from build123d import *

# Parameters (mm, degrees)
F0_W     = 40
F0_H     = 20
F0_W_2   = 80
F0_H_2   = 100
F0_R     = 5.444049
F0_H_3   = 20.000004
F0_R_2   = 5.262192
F0_R_3   = 5.424143
F1_DEPTH = 25


with BuildPart() as f1:
    # F0 (on Front) → F1 (new body)
    with BuildSketch(Plane.XZ):
        Polygon((-162.994809, -39.040719), (-162.994809, -53.924445), (-42.994809, -53.924445), (-42.994809, -33.45933), (-12.994809, -33.45933), (-12.994809, 66.540668), (-42.994809, 66.540668), (-42.994809, 86.075555), (-162.994809, 86.075555), (-162.994809, 76.773231), (-169.971554, 68.866255), (-212.994809, 68.866255), (-212.994809, -31.133745), (-169.971554, -31.133745), align=None)
        with Locations((-182.994809, -14.622118)):
            Rectangle(F0_W, F0_H, mode=Mode.SUBTRACT)
        with Locations((-104.85527, 13.749972)):
            Rectangle(F0_W_2, F0_H_2, mode=Mode.SUBTRACT)
        with Locations((-28.438857, -9.738397)):
            Circle(F0_R, mode=Mode.SUBTRACT)
        Polygon((-202.994809, 7.936021), (-202.994809, 27.936022), (-175.087825, 27.936022), (-162.994809, 27.936022), (-162.994809, 7.936021), (-175.087825, 7.936021), align=None, mode=Mode.SUBTRACT)
        with Locations((-182.994809, 49.563928)):
            Rectangle(F0_W, F0_H_3, mode=Mode.SUBTRACT)
        with Locations((-28.257, 21.424393)):
            Circle(F0_R_2, mode=Mode.SUBTRACT)
        with Locations((-28.418952, 48.866255)):
            Circle(F0_R_3, mode=Mode.SUBTRACT)
    extrude(amount=F1_DEPTH)


solid = f1.part
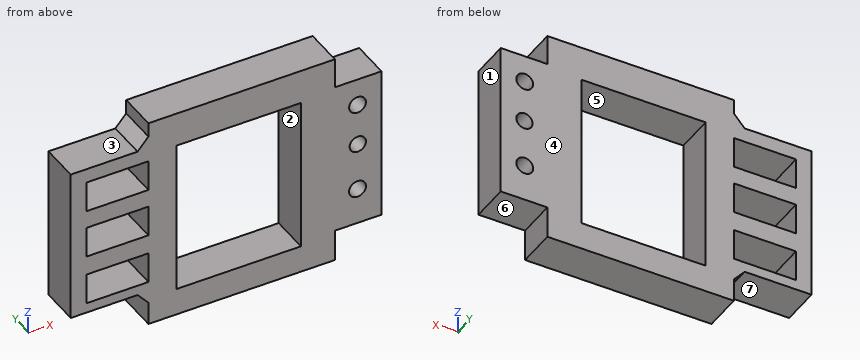
Here's how the part is built. I have some questions about the finished solid (model axes, mm). Face numbers are marked on the shaded views. A direction names the side the tool comes from. Round coordinates to 2 decimals unless told otherwise and drop trailing zeros. Write each loop counter-clockwise with the first axis right and the second up, starting at its lowest first coordinate (ties: lowest second). Pieces come first, ordered by that corner, then holes. Notation, with made-up numbers: (58, -17) -> (69, -17) arc R8 cw to (69, -7) -> close; hole circle Ø6 at (-0.75, 0.25). An arc over 180 degrees is marked (long way). One line per item, written item: value.
1) I'm going to push flat-ended pins straight in: pin 1 Ø7.5 at (x, y) = (-24, -8.5) entering from -Z; pin 2 Ø8 at (x, z) = (-142.5, -21.5) entering from -Y; pin 3 Ø3 at (x, y) = (-166.5, -2.5) entering from +Z; pin 4 Ø12.5 at (x, y) = (-191.5, -17.5) entering from +Z. Where does each tip first touch, or does it pass through?
Filled sheet:
pin 1: stops at z = -33.46
pin 2: stops at y = -25
pin 3: stops at z = 74.5
pin 4: stops at z = 68.87
2) Suppose I cut it at B-B on x = -142. List the corners of the cut face in (y, z) for me.
Filled sheet:
outline: (-25, -53.92) -> (0, -53.92) -> (0, -36.25) -> (-25, -36.25) -> close; (-25, 63.75) -> (0, 63.75) -> (0, 86.08) -> (-25, 86.08) -> close
3) We'd pull the mould along Z, two halves only. Please class the marked faces 1, 2 and 3: released by +Z, released by -Z, zero draft, split by the parting line, or undercut.
Filled sheet:
face 1: zero draft
face 2: undercut
face 3: released by +Z
4) If I drill on line 1 (X direction, y = -3.25, z = 13); line 2 (X direction, y = -8.5, z = 21.5); line 3 (Z direction, x = -199, y = -13), over which ranges is the centre line in solid material (lowest first)? Write a range as [from, to].
Filled sheet:
line 1: x = [-212.99, -202.99], [-162.99, -144.86], [-64.86, -12.99]
line 2: x = [-212.99, -202.99], [-162.99, -144.86], [-64.86, -33.52], [-23, -12.99]
line 3: z = [-31.13, -24.62], [-4.62, 7.94], [27.94, 39.56], [59.56, 68.87]
5) Suppose I cut it at C-C on y = -6. Give the number of separate pieces and of enclosed holes in the cut face, plus the area to 3 significant figures.
Filled sheet:
separate pieces: 1
enclosed holes: 7
area: 14,200 mm2
6) For the marked faces 4, 5, 6 and 7, which set-ups out of +Z, -Z, +X, -X, +Y, -Y let a thin tool reach every point of the face, with its end or its side?
Filled sheet:
face 4: +Z, -Z, +X, -X, +Y
face 5: +Y, -Y
face 6: -Z, +X, +Y, -Y
face 7: -Z, -X, +Y, -Y
7) Suppose I cut it at A-A on z = 0. List the corners of the cut face in (x, y) for me, plus the area to 3 significant figures.
Filled sheet:
outline: (-212.99, -25) -> (-144.86, -25) -> (-144.86, 0) -> (-212.99, 0) -> close; (-64.86, -25) -> (-12.99, -25) -> (-12.99, 0) -> (-64.86, 0) -> close
area: 3,000 mm2
